from build123d import *

# Parameters (mm, degrees)
SKETCH1_R                  = 6.35
BOSS_EXTRUDE1_DEPTH        = 233.9
F_10_24_TAPPED_HOLE1_D     = 3.7973
F_10_24_TAPPED_HOLE1_DEPTH = 12.83
F_10_24_TAPPED_HOLE1_TIP   = 1.140824014
F_10_24_TAPPED_HOLE2_D     = 3.7973
F_10_24_TAPPED_HOLE2_DEPTH = 12.83
F_10_24_TAPPED_HOLE2_TIP   = 1.140824014


with BuildPart() as part:
    # Sketch1 → Boss-Extrude1 (new body)
    with BuildSketch(Plane.XY):
        with Locations((110, 84.05)):
            Circle(SKETCH1_R)
    extrude(amount=-BOSS_EXTRUDE1_DEPTH)

    # #10-24 Tapped Hole1
    with Locations(Plane.XY):
        with Locations((110, 84.05)):
            Hole(F_10_24_TAPPED_HOLE1_D / 2, depth=F_10_24_TAPPED_HOLE1_DEPTH)
            with Locations((0, 0, -(F_10_24_TAPPED_HOLE1_DEPTH + F_10_24_TAPPED_HOLE1_TIP / 2))):  # 118° drill point
                Cone(0, F_10_24_TAPPED_HOLE1_D / 2, F_10_24_TAPPED_HOLE1_TIP, mode=Mode.SUBTRACT)

    # #10-24 Tapped Hole2
    with Locations(Plane(origin=(0, 0, -233.9), x_dir=(-1, 0, 0), z_dir=(0, 0, -1))):
        with Locations((-110, 84.05)):
            Hole(F_10_24_TAPPED_HOLE2_D / 2, depth=F_10_24_TAPPED_HOLE2_DEPTH)
            with Locations((0, 0, -(F_10_24_TAPPED_HOLE2_DEPTH + F_10_24_TAPPED_HOLE2_TIP / 2))):  # 118° drill point
                Cone(0, F_10_24_TAPPED_HOLE2_D / 2, F_10_24_TAPPED_HOLE2_TIP, mode=Mode.SUBTRACT)


solid = part.part
Read the model definition and answer for the solid it produces. Units are mm, in the model's axes. A direction names the side the tool comes from. Coordinates: 2 decimals unless noted, no trailing zeros. Loops run counter-clockwise (first coordinate to the right, second up) from the corner with the lowest first, then second, coordinate; pieces in that order, holes last.
Q1. The part is cut by section B-B on y = 88.5. Write down the section's boundary in (x, z).
Q2. The part is cut by section C-C on y = 80. Write down the section's boundary in (x, z), and give its area (3 significant figures).
Q3. Each of these flat-tipped pins is pushed along its axis until it touches: pin 1 Ø4 at (y, z) = (87.5, -110) entering from +X; pin 2 Ø2 at (x, z) = (112, -129) entering from -Y; pin 3 Ø1 at (y, z) = (88.5, -205) entering from +X. Where does it stop, or does it pass through?
Q4. The mould has two halves that part along Y. Classify faces 1 (the face through (113.414, 89.404, -115.313)), 2 (the face through (110.305, 83.924, -13.773)), 3 (the face through (108, 83, -233.9)): +Y half, -Y half, draft (parallel to the pull), parting line (faces both ways), or undercut.
Q5. Which of the six approach directions +Z, -Z, +X, -X, +Y, -Y give full straight-line access (tool end or side, diameter ignored) to faces 4 (the face through (108, 83, 0)), 5 (the face through (110.247, 85.932, -6.505)), 6 (the face through (109.753, 85.932, -227.395))?
Q6. The part is cut by section A-A on z = -140. Write down the section's boundary in (x, y).
Q7. Consider probe 1 along Y at (x, z) = (110, -9); probe 2 along X at (y, z) = (85.25, -10); probe 3 along Y at (x, z) = (114.75, -159.5). Determine where each line is inside the solid, lowest interval first.
Results below:
1. outline: (105.47, -233.9) - (114.53, -233.9) - (114.53, 0) - (105.47, 0) - close
2. outline: (105.11, -233.9) - (114.89, -233.9) - (114.89, 0) - (105.11, 0) - close
2. area: 2,290 mm2
3. pin 1: stops at x = 116.18
3. pin 2: stops at y = 77.78
3. pin 3: stops at x = 114.97
4. face 1: parting line
4. face 2: undercut
4. face 3: draft
5. face 4: +Z, +X, -X, +Y, -Y
5. face 5: +Z
5. face 6: -Z
6. outline: circle Ø12.7 at (110, 84.05)
7. probe 1: y = 77.7 to 82.15, 85.95 to 90.4
7. probe 2: x = 103.76 to 108.53, 111.47 to 116.24
7. probe 3: y = 79.84 to 88.26
